The listing builds one solid part. Answer for the finished solid, in the listing's coordinates (mm). Give positions to 0.01 mm unless a question says otherwise; leave off trailing zeros. Order: outer loops, then holes, each group sorted by start corner. A loop starts at its lowest first (then second) coordinate and runs counter-clockwise, first axis right, second up. Notation, with made-up numbers: (5.5, 72) - (33.5, 72) arc R28 cw to (33.5, 91) - close; hole circle Ø5 at (8.5, 7). An arc over 180 degrees is marked (long way). Answer in a Markdown table with one row per item.
from build123d import *

# Parameters (mm, degrees)
SKETCH1_W           = 13.8
SKETCH1_H           = 13.8
BOSS_EXTRUDE1_DEPTH = 3
SKETCH2_R           = 3.35
CUT_EXTRUDE1_DEPTH  = 4
CHAMFER1_SIZE       = 0.25
FILLET1_R           = 1
FILLET2_R           = 0.3


with BuildPart() as part:
    # Sketch1 → Boss-Extrude1 (new body)
    with BuildSketch(Plane(origin=(0, 0, 0), x_dir=(0, 0, -1), z_dir=(1, 0, 0))):
        Rectangle(SKETCH1_W, SKETCH1_H)
    extrude(amount=BOSS_EXTRUDE1_DEPTH)

    # Sketch2 → Cut-Extrude1 (cut, through all)
    with BuildSketch(Plane(origin=(0, 0, 0), x_dir=(0, 0, -1), z_dir=(1, 0, 0))):
        Circle(SKETCH2_R)
    extrude(amount=CUT_EXTRUDE1_DEPTH, mode=Mode.SUBTRACT)

    # Chamfer1
    chamfer1_edges = [part.edges().sort_by_distance(p)[0] for p in [
        (0, 0, 3.35),
        (3, 0, 3.35),
    ]]
    chamfer(chamfer1_edges, length=CHAMFER1_SIZE)

    # Fillet1
    fillet1_edges = [part.edges().sort_by_distance(p)[0] for p in [
        (1.5, 6.9, 6.9),
        (1.5, 6.9, -6.9),
        (1.5, -6.9, -6.9),
        (1.5, -6.9, 6.9),
    ]]
    fillet(fillet1_edges, radius=FILLET1_R)

    # Fillet2
    fillet2_edges = [part.edges().sort_by_distance(p)[0] for p in [
        (0, 6.9, 0),
        (3, 6.9, 0),
        (0, 0, 6.9),
        (0, 0, -6.9),
        (0, -6.9, 0),
        (0, 6.607106781, 6.607106781),
        (0, -6.607106781, 6.607106781),
        (0, -6.607106781, -6.607106781),
        (0, 6.607106781, -6.607106781),
        (3, 0, -6.9),
        (3, 0, 6.9),
        (3, -6.9, 0),
        (3, 6.607106781, 6.607106781),
        (3, -6.607106781, 6.607106781),
        (3, -6.607106781, -6.607106781),
        (3, 6.607106781, -6.607106781),
    ]]
    fillet(fillet2_edges, radius=FILLET2_R)


solid = part.part
Item 1: Determine the mould class of faces 1 (the face through (1.482, 0.147, 3.347)), 2 (the face through (1, 0, -6.9)), 3 (the face through (1.517, 6.599, 6.615)) for opening direction Y: pulls with the +Y half, pulls with the -Y half, needs draft (parallel to the pull), parting line crosses it, or undercut.
Answer block:
| item | result |
|---|---|
| face 1 | undercut |
| face 2 | needs draft |
| face 3 | pulls with the +Y half |
Item 2: Consider line 1 (Z direction, x = 1.6, y = 0); line 2 (Z direction, x = 2.45, y = -1.25). Determine where each line is inside the solid, lowest interval first.
Answer block:
| item | result |
|---|---|
| line 1 | -6.9 to -3.35, 3.35 to 6.9 |
| line 2 | -6.9 to -3.11, 3.11 to 6.9 |
Item 3: This flat-tipped pin is pushed along its axis until it touches: P1, Ø4, axis at y = -1, z = -1, coming from the -X side. Where does it stop, or does it pass through?
Answer block:
| item | result |
|---|---|
| P1 | x = 0.19 |
Item 4: Find section A-A on y = 0. Write down the section's boundary in (x, z), then the cut area to 3 significant figures.
Answer block:
| item | result |
|---|---|
| outline | (0, -6.6) arc R0.3 ccw to (0.3, -6.9) - (2.7, -6.9) arc R0.3 ccw to (3, -6.6) - (3, -3.6) - (2.75, -3.35) - (0.25, -3.35) - (0, -3.6) - close; (0, 3.6) - (0.25, 3.35) - (2.75, 3.35) - (3, 3.6) - (3, 6.6) arc R0.3 ccw to (2.7, 6.9) - (0.3, 6.9) arc R0.3 ccw to (0, 6.6) - close |
| area | 21.1 mm² |
Item 5: Find section C-C on x = 1.05. Write down the section's boundary in (y, z).
Answer block:
| item | result |
|---|---|
| outline | (-6.9, -5.9) arc R1 ccw to (-5.9, -6.9) - (5.9, -6.9) arc R1 ccw to (6.9, -5.9) - (6.9, 5.9) arc R1 ccw to (5.9, 6.9) - (-5.9, 6.9) arc R1 ccw to (-6.9, 5.9) - close; hole circle Ø6.7 at (0, 0) |
